Here's the drawing with two shaded views (mm, measured from the low corner). I have some questions. A direction names the side the tool comes from. Coordinates: 2 decimals unless noted, no trailing zeros. Write each loop counter-clockwise with the first axis right and the second up, starting at its lowest first coordinate (ties: lowest second). Pieces come first, ordered by that corner, then holes. Notation, with made-up numbers: (4.5, 49.5) -> (46.5, 49.5) arc R20 cw to (46.5, 57.5) -> close; hole circle Ø11 at (24.25, 71). An arc over 180 degrees is marked (long way). Use a Markdown table: item, result. Add a question column.
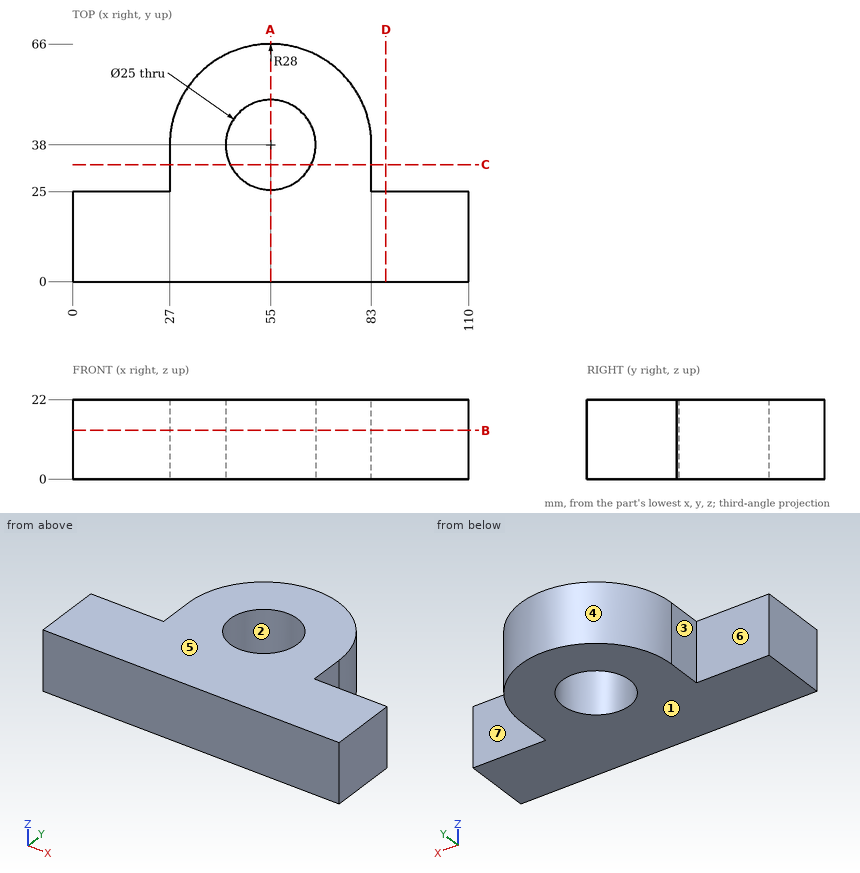
Q1. Suppose I cut it at D-D, the plane x = 87. Write out the boundary of the cut face in (y, z).
Q2. Suppose I cut it at A-A, the plane x = 55. Write out the boundary of the cut face in (y, z).
Q3. Thinking about a two-plate mould opening in X: for the marked faces 1, 2, 3 and 4, which applies, released by +X, released by -X, zero draft, split by the parting line, or undercut?
Q4. Suppose I cut it at B-B, the plane z = 13.5. Write out the boundary of the cut face in (x, y).
Q5. Which directions (+Z, -Z, +X, -X, +Y, -Y) give clear straight access to the entire face, cutting with the end or side of a thin tool? Please do the marked faces 5, 6 and 7.
Q6. Please list where these lines run through material, in increasing order: line 1 (Y direction, x = 55, z = 6.5); line 2 (Y direction, x = 105, z = 12.75); line 3 (X direction, y = 36, z = 20.25).
Q7. Will these pins go through, and if not, where does the flat tip stop? pin 1 (22.5 mm diameter, centred on x = 55, y = 38, fed in from -Z); pin 2 (1.5 mm diameter, centred on x = 55, z = 8, fed in from +Y); pin 3 (11 mm diameter, centred on x = 100.5, z = 12.5, fed in from +Y); pin 4 (1 mm diameter, centred on y = 39.5, z = 6, fed in from +X).
Q8. Suppose I cut it at C-C, the plane y = 32.5. Write out the boundary of the cut face in (x, z), and give its area (3 significant figures).
Answer key:
| question | item | result |
|---|---|---|
| 1 | outline | (0, 0) -> (25, 0) -> (25, 22) -> (0, 22) -> close |
| 2 | outline | (0, 0) -> (25.5, 0) -> (25.5, 22) -> (0, 22) -> close; (50.5, 0) -> (66, 0) -> (66, 22) -> (50.5, 22) -> close |
| 3 | face 1 | zero draft |
| 3 | face 2 | undercut |
| 3 | face 3 | released by -X |
| 3 | face 4 | split by the parting line |
| 4 | outline | (0, 0) -> (110, 0) -> (110, 25) -> (83, 25) -> (83, 38) arc R28 ccw to (27, 38) -> (27, 25) -> (0, 25) -> close; hole circle Ø25 at (55, 38) |
| 5 | face 5 | +Z, +X, -X, +Y, -Y |
| 5 | face 6 | +Z, -Z, -X, +Y |
| 5 | face 7 | +Z, -Z, +X, +Y |
| 6 | line 1 | y = 0 to 25.5, 50.5 to 66 |
| 6 | line 2 | y = 0 to 25 |
| 6 | line 3 | x = 27 to 42.66, 67.34 to 83 |
| 7 | pin 1 | passes through |
| 7 | pin 2 | stops at y = 66 |
| 7 | pin 3 | stops at y = 25 |
| 7 | pin 4 | stops at x = 82.98 |
| 8 | outline | (27, 0) -> (43.78, 0) -> (43.78, 22) -> (27, 22) -> close; (66.22, 0) -> (83, 0) -> (83, 22) -> (66.22, 22) -> close |
| 8 | area | 738 mm^2 |
